The drawing under review shows one solid part. Ordinate dimensions are in mm from its lowest x, y, z. A direction names the side the tool comes from. Round coordinates to 2 decimals unless told otherwise and drop trailing zeros. Write each loop counter-clockwise with the first axis right and the second up, starting at its lowest first coordinate (ties: lowest second). Pieces come first, ordered by that corner, then holes. Notation, with made-up numbers: M 45.25,-38.5 L 52.25,-38.5 A12 cw 52.25,-34.5 Z; hole C 81,57 d7. An arc over 180 degrees is marked long. Write item = value, one per line. Start each with the question number.
Item 1: To check wall thickness, follow line 1 along X through (y, z) = (6.75, 13.85); line 2 along Y through (x, z) = (10.5, 10.5); line 3 along Y through (x, z) = (16, 23). State the ranges of each line that lie inside material, in increasing order.
Item 2: Take a section at A-A, the plane x = 13.85. Give the boundary of the cut face in (y, z).
Item 3: For pin 1 Ø3 at (x, z) = (13.85, 19.85) entering from +Y; pin 2 Ø6 at (x, y) = (5, 7.5) entering from +Z; pin 3 Ø2.5 at (x, z) = (21.85, 13.85) entering from +Y; pin 4 Ø3 at (y, z) = (19, 18) entering from +X, all flat-tipped, find the tip position at first contact; note any pin that passes through.
Item 4: Take a section at B-B, the plane z = 13.85. Give the boundary of the cut face in (x, y).
Item 5: Take a section at C-C, the plane y = 9.75. Give the boundary of the cut face in (x, z), plus the area to 3 significant figures.
Item 6: Tool access review of the marked faces 1 and 2: name each direction out of +Z, -Z, +X, -X, +Y, -Y from which nothing blocks a thin tool from reaching the whole face with its end or side.
Item 7: Take a section at D-D, the plane y = 24.25. Give the boundary of the cut face in (x, z), plus the area to 3 significant figures.
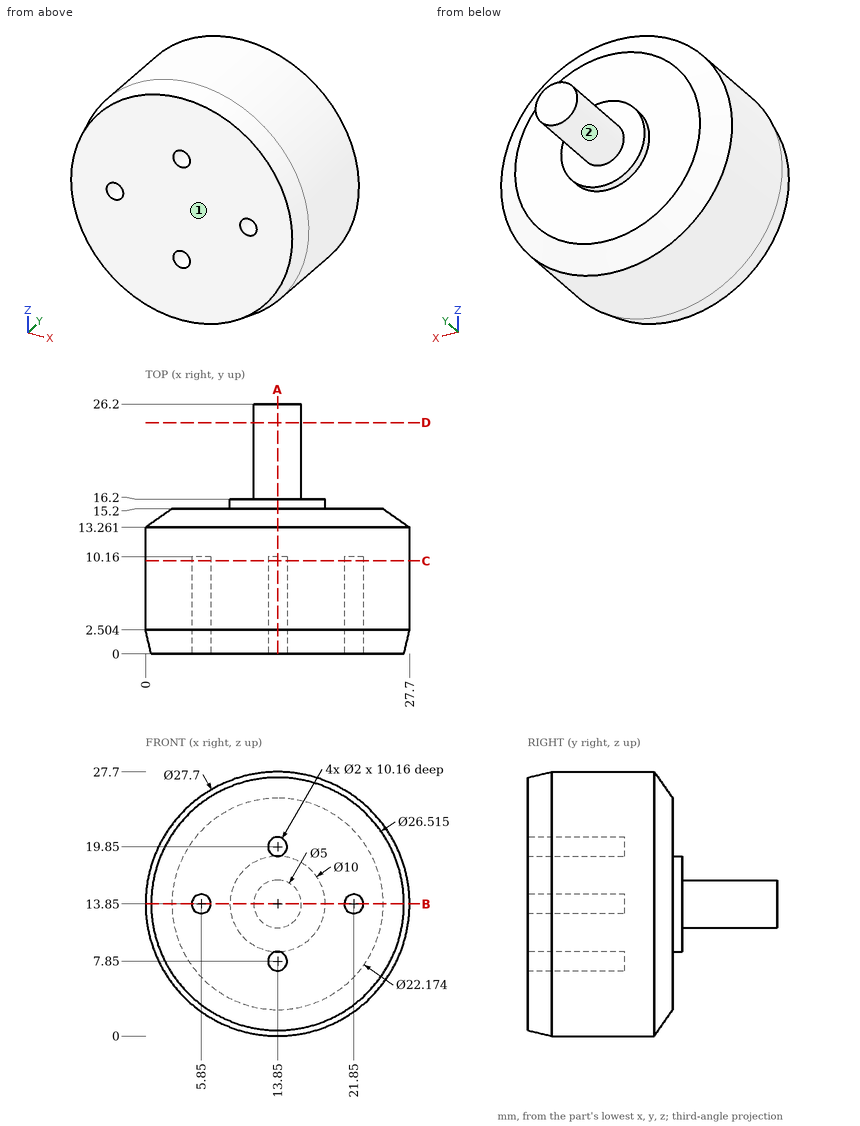
Response values:
q1.line_1 = 0 to 4.85, 6.85 to 20.85, 22.85 to 27.7
q1.line_2 = 0 to 16.2
q1.line_3 = 0 to 15.2
q2.outline = M 0,0.59 L 2.5,0 L 13.26,0 L 15.2,2.76 L 15.2,8.85 L 16.2,8.85 L 16.2,11.35 L 26.2,11.35 L 26.2,16.35 L 16.2,16.35 L 16.2,18.85 L 15.2,18.85 L 15.2,24.94 L 13.26,27.7 L 2.5,27.7 L 0,27.11 L 0,20.85 L 10.16,20.85 L 10.16,18.85 L 0,18.85 L 0,8.85 L 10.16,8.85 L 10.16,6.85 L 0,6.85 Z
q3.pin_1 = 16.2
q3.pin_2 = 26.4
q3.pin_3 = 15.2
q3.pin_4 = through
q4.outline = M 0,2.5 L 0.59,0 L 4.85,0 L 4.85,10.16 L 6.85,10.16 L 6.85,0 L 20.85,0 L 20.85,10.16 L 22.85,10.16 L 22.85,0 L 27.11,0 L 27.7,2.5 L 27.7,13.26 L 24.94,15.2 L 18.85,15.2 L 18.85,16.2 L 16.35,16.2 L 16.35,26.2 L 11.35,26.2 L 11.35,16.2 L 8.85,16.2 L 8.85,15.2 L 2.76,15.2 L 0,13.26 Z
q5.outline = C 13.85,13.85 d27.7; hole C 5.85,13.85 d2; hole C 13.85,7.85 d2; hole C 13.85,19.85 d2; hole C 21.85,13.85 d2
q5.area = 590 mm2
q6.face_1 = +Z, -Z, +X, -X, -Y
q6.face_2 = +Y
q7.outline = C 13.85,13.85 d5
q7.area = 19.6 mm2
